The listing builds one solid part. Answer for the finished solid, in the listing's coordinates (mm). Face numbers are marked on the shaded views. A direction names the side the tool comes from. Coordinates: 2 decimals unless noted, no trailing zeros. Write each loop counter-clockwise with the first axis right and the second up, starting at its lowest first coordinate (ties: lowest second). Pieces come first, ordered by that corner, then holes. Notation, with made-up numbers: M 85,58 L 105,58 A11 ccw 105,65 Z; hole C -34.75,6 d2. An arc over 180 degrees is marked long. Answer as CSV lines item,"result". Start each with the question number.
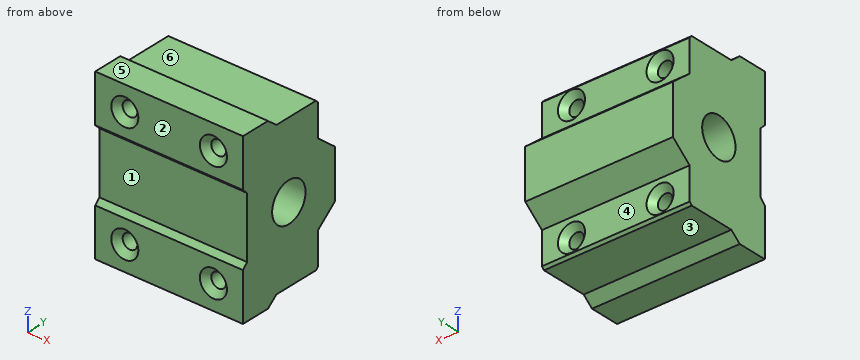
Autodesk Inventor part; units mm, degrees
ref_plane "YZ Plane" through (0, 0, 0) normal (1, 0, 0) x (0, 1, 0)
ref_plane "XZ Plane" through (0, 0, 0) normal (0, 1, 0) x (-1, 0, 0)
ref_plane "XY Plane" through (0, 0, 0) normal (0, 0, 1) x (1, 0, 0)
sketch "Sketch1" plane through (0, 0, 0) normal (1, 0, 0) x (0, 1, 0)
  line L0 (14.2461, 0) -> (-14.2461, 0) construction
  line L1 (11, 5) -> (11, -5)
  line L2 (11, -5) -> (7, -8.3)
  line L3 (7, -8.3) -> (7, -15.35)
  line L4 (7, -15.35) -> (-3, -15.35)
  line L5 (-3, -15.35) -> (-5, -17)
  line L6 (-5, -17) -> (-11, -17)
  line L7 (-11, 17) -> (-5, 17)
  line L8 (-5, 17) -> (-3, 15.35)
  line L9 (-3, 15.35) -> (7, 15.35)
  line L10 (7, 15.35) -> (7, 8.3)
  line L11 (7, 8.3) -> (11, 5)
  line L12 (-11, -17) -> (-11, -7.25)
  line L13 (-11, -7.25) -> (-10, -6.25)
  line L14 (-10, -6.25) -> (-10, 6.25)
  line L15 (-10, 6.25) -> (-11, 7.25)
  line L16 (-11, 7.25) -> (-11, 17)
  circle A0 centre (0, 0) radius 4
  point P0 (-11, -12.125)
  dimension "d2" = 45
  dimension "d3" = 22
  dimension "d4" = 34
  dimension "d5" = 6
  dimension "d6" = 8
  dimension "d7" = 11
  dimension "d8" = 8
  dimension "d9" = 18
  dimension "d10" = 16.6
  dimension "d11" = 12.5
  dimension "d12" = 1
  dimension "d13" = 10
extrude "Extrusion1" add sketch "Sketch1" along normal mid plane 30
sketch "Sketch2" plane through (-15, 7, 15.35) normal (0, 1, 0) x (1, 0, 0)
  line L0 (-4.3659, 15.35) -> (34.0137, 15.35) construction
  line L1 (0, 10.35) -> (0, 20.35)
  line L2 (0, 10.35) -> (30, 10.35)
  line L3 (15, 2.4961) -> (15, 28.0168) construction
  point P0 (15, 15.35)
  point P1 (6, 3.35)
  point P2 (6, 27.35)
  point P3 (24, 27.35)
  point P4 (24, 3.35)
  point P5 (0, 15.35)
  point P6 (15, 10.35)
  dimension "d16" = 24
  dimension "d17" = 18
hole "Hole1" at (-9, 7, 12) at (-9, 7, -12) at (9, 7, -12) at (9, 7, 12) direction (0, -1, 0) diameter 3 depth 8 countersink diameter 5.5 countersink angle 90
sketch "Sketch3" plane through (-15, -11, 7.25) normal (0, -1, 0) x (1, 0, 0)
  point P0 (15, -7.25)
  point P1 (6, 4.75)
  point P2 (24, 4.75)
  point P3 (6, -19.25)
  point P4 (24, -19.25)
hole "Hole2" at (-9, -11, 12) at (9, -11, 12) at (-9, -11, -12) at (9, -11, -12) direction (0, 1, 0) diameter 3 end through all countersink diameter 5.5 countersink angle 90
chamfer "Chamfer1" distance 0.5 angle 45 2 edges at (0, 7, 15.35) (0, 7, -15.35)
properties part number "Bearing block"
1) For a pull along Z with two mould halves and no side action, classify the marked faces 1, 2 and 3 as +Z half, -Z half, draft (parallel to the pull), parting line (faces both ways), or undercut.
2) The part is cut by section A-A (z = 0). Determine the outline of the cut face in (x, y), then the cut area to 3 significant figures.
3) The part is cut by section B-B (y = -7.75). Determine the outline of the cut face in (x, z), then the cut area to 3 significant figures.
4) Which of the six approach directions +Z, -Z, +X, -X, +Y, -Y give full straight-line access (tool end or side, diameter ignored) to the marked faces 4, 5 and 6?
5) Find the intervals of material crossed by line 1 (X direction, y = -5, z = 12); line 2 (Z direction, x = -9, y = -5.5); line 3 (Z direction, x = -9, y = -3.5), in increasing order. Write a range as from..to.
6) Each of these flat-tipped pins is pushed along its axis until it touches: P1, Ø3, axis at x = -12, y = 4, coming from the +Z side; P2, Ø10.5, axis at x = 1, y = 0.5, coming from the +Z side; P3, Ø3.5, axis at x = 2.5, z = 11, coming from the +Y side. Where does it stop, or does it pass through?
7) The part is cut by section D-D (x = 12.25). Determine the outline of the cut face in (y, z), then the cut area to 3 significant figures.
8) The part is cut by section C-C (y = 0). Determine the outline of the cut face in (x, z).
Completed:
1,face 1,"undercut"
1,face 2,"draft"
1,face 3,"-Z half"
2,outline,"M -15,-10 L 15,-10 L 15,-4 L -15,-4 Z; M -15,4 L 15,4 L 15,11 L -15,11 Z"
2,area,"390 mm²"
3,outline,"M -15,-17 L 15,-17 L 15,17 L -15,17 Z; hole C -9,-12 d3; hole C -9,12 d3; hole C 9,-12 d3; hole C 9,12 d3"
3,area,"992 mm²"
4,face 4,"-Z, +X, -X, +Y"
4,face 5,"+Z, +X, -X, +Y, -Y"
4,face 6,"+Z, +X, -X, +Y"
5,line 1,"-15..-10.5, -7.5..7.5, 10.5..15"
5,line 2,"-17..-13.5, -10.5..10.5, 13.5..17"
5,line 3,"-15.76..-13.5, -10.5..-1.94, 1.94..10.5, 13.5..15.76"
6,P1,"z = 15.35"
6,P2,"z = 16.79"
6,P3,"y = 7"
7,outline,"M -11,-17 L -5,-17 L -3,-15.35 L 6.5,-15.35 L 7,-14.85 L 7,-8.3 L 11,-5 L 11,5 L 7,8.3 L 7,14.85 L 6.5,15.35 L -3,15.35 L -5,17 L -11,17 L -11,7.25 L -10,6.25 L -10,-6.25 L -11,-7.25 Z; hole C 0,0 d8"
7,area,"565 mm²"
8,outline,"M -15,-15.35 L 15,-15.35 L 15,-4 L -15,-4 Z; M -15,4 L 15,4 L 15,15.35 L -15,15.35 Z; hole C -9,-12 d3; hole C -9,12 d3; hole C 9,-12 d3; hole C 9,12 d3"
